Verification items for the finished model (mm, model axes). A direction names the side the tool comes from. Coordinates: 2 decimals unless noted, no trailing zeros. Write each loop counter-clockwise with the first axis right and the second up, starting at its lowest first coordinate (ties: lowest second). Pieces come first, ordered by that corner, then holes. Notation, with made-up numbers: M 36,8.5 L 61,8.5 A21 ccw 61,44.5 Z; hole C 10.25,21 d2. An arc over 180 degrees is marked long. One line per item, written item: value.
```python
from build123d import *

# Parameters (mm, degrees)
SKETCH1_W                = 15
SKETCH1_H                = 13.5
BOSS_EXTRUDE1_DEPTH      = 10
FILLET1_R                = 2
M5_PORTS_D               = 4.2
M5_PORTS_DEPTH           = 5
M5_PORTS_ON_FACE_2_D     = 4.2
M5_PORTS_ON_FACE_2_DEPTH = 5
M5_PORT_CHAMFER_SIZE     = 0.25
SKETCH3_R                = 1.25
CUT_EXTRUDE1_DEPTH       = 4
CHAMFER2_SIZE            = 0.15


with BuildPart() as part:
    # Sketch1 → Boss-Extrude1 (new, symmetric)
    with BuildSketch(Plane.XY):
        with Locations((0, 0.75)):
            Rectangle(SKETCH1_W, SKETCH1_H)
    extrude(amount=BOSS_EXTRUDE1_DEPTH, both=True)

    # Fillet1
    fillet1_edges = [part.edges().sort_by_distance(p)[0] for p in [
        (-7.5, 0.75, 10),
        (7.5, 0.75, 10),
        (-7.5, 0.75, -10),
        (7.5, 0.75, -10),
    ]]
    fillet(fillet1_edges, radius=FILLET1_R)

    # M5 Ports
    with Locations(Plane.XY.offset(10)):
        with Locations((0, 0)):
            Hole(M5_PORTS_D / 2, depth=M5_PORTS_DEPTH)

    # M5 Ports on face 2
    with Locations(Plane(origin=(0, 0, -10), x_dir=(-1, 0, 0), z_dir=(0, 0, -1))):
        with Locations((0, 0)):
            Hole(M5_PORTS_ON_FACE_2_D / 2, depth=M5_PORTS_ON_FACE_2_DEPTH)

    # M5 Port Chamfer
    m5_port_chamfer_edges = [part.edges().sort_by_distance(p)[0] for p in [
        (-2.1, 0, -10),
        (2.1, 0, 10),
    ]]
    chamfer(m5_port_chamfer_edges, length=M5_PORT_CHAMFER_SIZE)

    # Sketch3 → Cut-Extrude1 (cut)
    with BuildSketch(Plane.XZ.offset(6)):
        with Locations(Location((-5.5, 0, 0), (0, 0, 270))):
            Circle(SKETCH3_R)
        with Locations(Location((5.5, 0, 0), (0, 0, 270))):
            Circle(SKETCH3_R)
    extrude(amount=-CUT_EXTRUDE1_DEPTH, mode=Mode.SUBTRACT)

    # Chamfer2
    chamfer2_edges = [part.edges().sort_by_distance(p)[0] for p in [
        (-5.5, -6, 1.25),
        (5.5, -6, 1.25),
    ]]
    chamfer(chamfer2_edges, length=CHAMFER2_SIZE)


solid = part.part
```
Item 1: Cross-section at A-A, the plane y = -4.25. Enter the section's corners in (x, z).
The answers:
outline: M -7.5,-8 A2 ccw -5.5,-10 L 5.5,-10 A2 ccw 7.5,-8 L 7.5,8 A2 ccw 5.5,10 L -5.5,10 A2 ccw -7.5,8 Z; hole C -5.5,0 d2.5; hole C 5.5,0 d2.5
Item 2: Cross-section at D-D, the plane y = 0. Enter the section's corners in (x, z), and give its area (3 significant figures).
The answers:
outline: M -7.5,-8 A2 ccw -5.5,-10 L -2.35,-10 L -2.1,-9.75 L -2.1,-5 L 2.1,-5 L 2.1,-9.75 L 2.35,-10 L 5.5,-10 A2 ccw 7.5,-8 L 7.5,8 A2 ccw 5.5,10 L 2.35,10 L 2.1,9.75 L 2.1,5 L -2.1,5 L -2.1,9.75 L -2.35,10 L -5.5,10 A2 ccw -7.5,8 Z
area: 254 mm²
Item 3: Cross-section at C-C, the plane x = 0. Enter the section's corners in (y, z).
The answers:
outline: M -6,-10 L -2.35,-10 L -2.1,-9.75 L -2.1,-5 L 2.1,-5 L 2.1,-9.75 L 2.35,-10 L 7.5,-10 L 7.5,10 L 2.35,10 L 2.1,9.75 L 2.1,5 L -2.1,5 L -2.1,9.75 L -2.35,10 L -6,10 Z
Item 4: Cross-section at B-B, the plane z = -5.25. Enter the section's corners in (x, y), and give its area (3 significant figures).
The answers:
outline: M -7.5,-6 L 7.5,-6 L 7.5,7.5 L -7.5,7.5 Z; hole C 0,0 d4.2
area: 189 mm²
Item 5: Scan lines: line 1 (X direction, y = -4.15, z = 0); line 2 (Y direction, x = 0, z = 6.35); line 3 (Y direction, x = -4.75, z = 0.25). Record each from-to range of solid material in increasing order.
The answers:
line 1: x = -7.5 to -6.75, -4.25 to 4.25, 6.75 to 7.5
line 2: y = -6 to -2.1, 2.1 to 7.5
line 3: y = -2 to 7.5
Item 6: Access from +Z, -Z, +X, -X, +Y, -Y to the whole of each face (thin tool, end or side, straight path). Record for faces 5 (the face through (6, -2, 0)), 6 (the face through (0, 0, -5)), 7 (the face through (0, 0, 5)).
The answers:
face 5: -Y
face 6: -Z
face 7: +Z
Item 7: Draft check along Z on faces 1 (the face through (-6.93, 0.84, -9.4)), 2 (the face through (2.003, 0.631, -7.342)), 3 (the face through (-1.3, 2.3, 10)), 4 (the face through (4.28, -3.95, 0.27)). Enter one of: released by +Z, released by -Z, zero draft, split by the parting line, or undercut.
The answers:
face 1: released by -Z
face 2: zero draft
face 3: released by +Z
face 4: undercut
Item 8: Go/stop test with flat-tipped pins: P1, Ø3.5, axis at x = 0, y = 0, coming from the -Z side; P2, Ø4, axis at x = 0, y = 0, coming from the +Z side. Record where each tip stops, or that it passes through.
The answers:
P1: stops at z = -5
P2: stops at z = 5
